Autodesk Inventor part; units mm, degrees
ref_plane "YZ Plane" through (0, 0, 0) normal (1, 0, 0) x (0, 1, 0)
ref_plane "XZ Plane" through (0, 0, 0) normal (0, 1, 0) x (-1, 0, 0)
ref_plane "XY Plane" through (0, 0, 0) normal (0, 0, 1) x (1, 0, 0)
sketch "Sketch1" plane through (0, 0, 0) normal (0, 0, 1) x (1, 0, 0)
  line L0 (0, 0) -> (113.5126, 0)
  line L1 (0, 2.3813) -> (3.9624, 2.3813)
  line L2 (3.9624, 2.3813) -> (3.9624, 0)
  line L3 (0, 0) -> (0, 2.3813)
  line L4 (0, 0) -> (0, 11.1125)
  line L5 (6.35, 17.4625) -> (107.1626, 17.4625)
  line L6 (0, 17.4625) -> (0, 11.1125)
  line L7 (3.9624, 11.1125) -> (113.5126, 11.1125)
  line L8 (0, 17.4625) -> (3.9624, 17.4625)
  line L9 (3.9624, 11.1125) -> (3.9624, 2.3813)
  arc A0 (6.35, 17.4625) -> (0, 11.1125) centre (6.35, 11.1125) ccw
  line L10 (113.5126, 11.1125) -> (113.5126, 11.1125)
  arc A1 (113.5126, 11.1125) -> (107.1626, 17.4625) centre (107.1626, 11.1125) ccw
  point P0 (113.5126, 17.4625)
  dimension "d0" = 113.5126
  dimension "d1" = 2.3813
  dimension "d2" = 3.9624
  dimension "d3" = 17.4625
  dimension "d4" = 113.5126
  dimension "d5" = 6.35
  dimension "d6" = 113.5126
  dimension "d7" = 3.9624
  dimension "d8" = 6.35
  dimension "d9" = 6.35
revolve "Revolution1" add sketch "Sketch1" angle 360 about axis through (0, 0, 0) along (1, 0, 0) contours L4 A0 L5 A1 L7 L9 L1
properties part number "Rubber Sleeve"
Read the model definition and answer for the solid it produces. Units are mm, in the model's axes. Round coordinates to 2 decimals unless told otherwise and drop trailing zeros. Write each loop counter-clockwise with the first axis right and the second up, starting at its lowest first coordinate (ties: lowest second). Pieces come first, ordered by that corner, then holes.
Q1. The mould has two halves that part along Z. Classify faces 1 (the face through (0, -3, 0)), 2 (the face through (2.01, 1.1, -2.11)), 3 (the face through (57.462, -13.858, -10.626)): released by +Z, released by -Z, zero draft, split by the parting line, or undercut.
Values:
face 1: zero draft
face 2: undercut
face 3: split by the parting line
Q2. Find section A-A on y = 0. Determine the outline of the cut face in (x, z), and give its area (3 significant figures).
Values:
outline: (0, -11.11) arc R6.35 ccw to (6.35, -17.46) - (107.16, -17.46) arc R6.35 ccw to (113.51, -11.11) - (3.96, -11.11) - (3.96, -2.38) - (0, -2.38) - close; (0, 2.38) - (3.96, 2.38) - (3.96, 11.11) - (113.51, 11.11) arc R6.35 ccw to (107.16, 17.46) - (6.35, 17.46) arc R6.35 ccw to (0, 11.11) - close
area: 1,480 mm2
Q3. Straight lines are drawn through the part: line 1 (Z direction, x = 60, y = 0); line 2 (Y direction, x = 88, z = -10); line 3 (X direction, y = -6.5, z = -4.5). For each, find the intervals that lie inside material, in ascending order.
Values:
line 1: z = -17.46 to -11.11, 11.11 to 17.46
line 2: y = -14.32 to -4.85, 4.85 to 14.32
line 3: x = 0 to 3.96
Q4. Find section C-C on x = 87. Determine the outline of the cut face in (y, z) (1 decimal).
Values:
outline: circle Ø34.9 at (0, 0); hole circle Ø22.2 at (0, 0)
Q5. Flat-ended cylindrical pins translate along their axes: P1, Ø12, axis at x = 44.5, y = 9, coming from the +Z side; P2, Ø4, axis at y = -6, z = -3, coming from the +X side; P3, Ø3, axis at y = 13.5, z = -8, coming from the -X side. Find the tip coordinate at first contact, or state that the pin passes through.
Values:
P1: stops at z = 17.2
P2: stops at x = 3.96
P3: stops at x = 0.8
